```python
from build123d import *

# Parameters (mm, degrees)
RC_START                                     = -6.5
SKETCH1_R                                    = 4.4
RC_1_8_CONNECTION_THREAD_CORE_ENVELOPE_DEPTH = 6.5
SKETCH2_W                                    = 12
SKETCH2_H                                    = 12
ELBOW_BODY_AND_12_MM_WRENCH_FLATS_DEPTH      = 18
MALE_START                                   = 5.8
SKETCH3_R                                    = 5.55
MALE_4_JIC_OUTLET_ENVELOPE_DEPTH             = 13.7


with BuildPart() as part:
    # Sketch1 → Rc 1/8 connection, thread core envelope (new body)
    with BuildSketch(Plane.XY.offset(RC_START)):
        with Locations(Location((0, 0, 0), (0, 0, 180))):
            Circle(SKETCH1_R)
    extrude(amount=RC_1_8_CONNECTION_THREAD_CORE_ENVELOPE_DEPTH)

    # Sketch2 → Elbow body and 12 mm wrench flats (add)
    with BuildSketch(Plane.XY):
        Rectangle(SKETCH2_W, SKETCH2_H)
    extrude(amount=ELBOW_BODY_AND_12_MM_WRENCH_FLATS_DEPTH)

    # Sketch3 → Male -4 JIC outlet envelope (add)
    with BuildSketch(Plane(origin=(0, 0, 0), x_dir=(0, 0, -1), z_dir=(1, 0, 0)).offset(MALE_START)):
        with Locations(Location((-12, 0, 0), (0, 0, 180))):
            Circle(SKETCH3_R)
    extrude(amount=MALE_4_JIC_OUTLET_ENVELOPE_DEPTH)


solid = part.part
```
Part model, mm, in its own coordinate system. A direction names the side the tool comes from. Coordinates: 2 decimals unless noted, no trailing zeros. Write each loop counter-clockwise with the first axis right and the second up, starting at its lowest first coordinate (ties: lowest second). Pieces come first, ordered by that corner, then holes.
Item 1: Which spindle directions (+Z, -Z, +X, -X, +Y, -Y) get a long thin tool onto all of the face, cutting with end or side? Do faces 1 (the face through (6, 0, 5)), 2 (the face through (0, 0, -6.5)), 3 (the face through (3, 4, 0)). Say none if no direction does.
Item 2: Slice it at C-C (y = 1.5). Write the cut outline in (x, z).
Item 3: Slice it at D-D (y = 4). Write the cut outline in (x, z).
Item 4: Probe line 1 (Z direction, x = -3.5, y = -5); line 2 (X direction, y = -1.75, z = 2.25); line 3 (Z direction, x = 17.25, y = 4.75). List the from-to ranges inside material, lowest first.
Item 5: Slice it at B-B (z = 12). Write the cut outline in (x, y).
Item 6: Slice it at A-A (x = 0). Write the cut outline in (y, z).
Item 7: Pin check, flat tip, straight feed: pin 1 (8 mm diameter, centred on x = 15.5, z = 7.5, fed in from +Y). Stop position of the tip, or through.
Results found:
1. face 1: +X
1. face 2: -Z, +X, -X, +Y, -Y
1. face 3: -Z
2. outline: (-6, 0) - (-4.14, 0) - (-4.14, -6.5) - (4.14, -6.5) - (4.14, 0) - (6, 0) - (6, 6.66) - (19.5, 6.66) - (19.5, 17.34) - (6, 17.34) - (6, 18) - (-6, 18) - close
3. outline: (-6, 0) - (-1.83, 0) - (-1.83, -6.5) - (1.83, -6.5) - (1.83, 0) - (6, 0) - (6, 8.15) - (19.5, 8.15) - (19.5, 15.85) - (6, 15.85) - (6, 18) - (-6, 18) - close
4. line 1: z = 0 to 18
4. line 2: x = -6 to 6
4. line 3: z = 9.13 to 14.87
5. outline: (-6, -6) - (6, -6) - (6, -5.55) - (19.5, -5.55) - (19.5, 5.55) - (6, 5.55) - (6, 6) - (-6, 6) - close
6. outline: (-6, 0) - (-4.4, 0) - (-4.4, -6.5) - (4.4, -6.5) - (4.4, 0) - (6, 0) - (6, 18) - (-6, 18) - close
7. pin 1: stops at y = 5.53
